```python
from build123d import *

# Parameters (mm, degrees)
SKETCH1_R           = 50
BOSS_EXTRUDE1_DEPTH = 10
SKETCH2_R           = 72.5
CUT_EXTRUDE1_DEPTH  = 352.523431325


with BuildPart() as part:
    # Sketch1 → Boss-Extrude1 (new body)
    with BuildSketch(Plane(origin=(0, 0, 0), x_dir=(0, 0, -1), z_dir=(1, 0, 0))):
        with BuildLine():
            ThreePointArc((81.153066922, 9.411970763), (0, 311.772037013), (-81.153066922, 9.411970763))
            ThreePointArc((-81.153066922, 9.411970763), (-67.666963002, -7.212746854), (-68.696324701, -28.59490412))
            ThreePointArc((-68.696324701, -28.59490412), (0, -133.691664287), (68.696324701, -28.59490412))
            ThreePointArc((68.696324701, -28.59490412), (67.666963002, -7.212746854), (81.153066922, 9.411970763))
        make_face()
        with Locations((0, 149.701312613)):
            Circle(SKETCH1_R, mode=Mode.SUBTRACT)
    extrude(amount=BOSS_EXTRUDE1_DEPTH)

    # Sketch2 → Cut-Extrude1 (cut, through all)
    with BuildSketch(Plane(origin=(10, 0, 0), x_dir=(0, 0, -1), z_dir=(1, 0, 0))):
        with Locations((0, -58.691664287)):
            Circle(SKETCH2_R)
    extrude(amount=-CUT_EXTRUDE1_DEPTH, mode=Mode.SUBTRACT)


solid = part.part
```
Work out the finished part from the listing and answer in its coordinate system (mm). Give positions to 0.01 mm unless a question says otherwise; leave off trailing zeros. Order: outer loops, then holes, each group sorted by start corner. A loop starts at its lowest first (then second) coordinate and runs counter-clockwise, first axis right, second up. Notation, with made-up numbers: (53, -25.5) - (76, -25.5) arc R21 ccw to (76, -19.5) - close; hole circle Ø10 at (60.25, 69.5). An arc over 180 degrees is marked (long way). One line per item, written item: value. Start each with the question number.
1. Consider line 1 (Y direction, x = 8.25, z = 0); line 2 (Y direction, x = 2.75, z = 23); line 3 (Z direction, x = 6.25, y = -4.5). Determine where each line is inside the solid, lowest interval first.
2. Section C-C, the plane z = -58.5 is taken. Write down the section's boundary in (x, y).
3. Section B-B, the plane y = 111.5 is taken. Write down the section's boundary in (x, z), then the cut area to 3 significant figures.
4. For a pull along Z with two mould halves and no side action, classify faces 1 (the face through (4.93, -6.922, 67.764)), 2 (the face through (5.07, 2.44, -38.98)), 3 (the face through (4.93, 100.89, 10.84)), 4 (the face through (0, 191, 38)) as released by +Z, released by -Z, zero draft, split by the parting line, or undercut.
5. Each of these flat-tipped pins is pushed along its axis until it touches: pin 1 Ø4 at (x, z) = (1, 81.5) entering from -Y; pin 2 Ø5 at (x, z) = (3.5, 82.5) entering from -Y; pin 3 Ø2 at (x, y) = (5.5, 168.5) entering from -Z. Where does it stop, or does it pass through?
6. Section A-A, the plane z = 0 is taken. Write down the section's boundary in (x, y), then the cut area to 3 significant figures.
7. Section D-D, the plane x = 6 is taken. Write down the section's boundary in (y, z), then the cut area to 3 significant figures.
Filled sheet:
1. line 1: -133.69 to -131.19, 13.81 to 99.7, 199.7 to 311.77
1. line 2: -130.08 to -127.45, 10.06 to 105.31, 194.1 to 310.13
1. line 3: -68.7 to -48.16, 48.16 to 68.7
2. outline: (0, -105.63) - (10, -105.63) - (10, -101.52) - (0, -101.52) - close; (0, -15.87) - (10, -15.87) - (10, 300.85) - (0, 300.85) - close
3. outline: (0, -157.5) - (10, -157.5) - (10, -32.26) - (0, -32.26) - close; (0, 32.26) - (10, 32.26) - (10, 157.5) - (0, 157.5) - close
3. area: 2,500 mm²
4. face 1: released by +Z
4. face 2: undercut
4. face 3: undercut
4. face 4: zero draft
5. pin 1: y = 8.38
5. pin 2: y = 8.71
5. pin 3: z = -161.09
6. outline: (0, -133.69) - (10, -133.69) - (10, -131.19) - (0, -131.19) - close; (0, 13.81) - (10, 13.81) - (10, 99.7) - (0, 99.7) - close; (0, 199.7) - (10, 199.7) - (10, 311.77) - (0, 311.77) - close
6. area: 2,000 mm²
7. outline: (-28.59, -68.7) arc R30 cw to (9.41, -81.15) arc R162.07 ccw (long way) to (9.41, 81.15) arc R30 cw to (-28.59, 68.7) arc R75 ccw (long way) to start; hole circle Ø145 at (-58.69, 0); hole circle Ø100 at (149.7, 0)
7. area: 74,300 mm²
